```python
from build123d import *

# Parameters (mm, degrees)
BOSS_EXTRUDE1_DEPTH = 100
FILLET1_R           = 10
SKETCH4_W           = 60
SKETCH4_H           = 8
CUT_EXTRUDE1_DEPTH  = 10
FILLET2_R           = 10
SKETCH5_W           = 12
SKETCH5_H           = 14
CUT_EXTRUDE2_DEPTH  = 10
CUT_EXTRUDE3_DEPTH  = 10


with BuildPart() as part:
    # Sketch1 → Boss-Extrude1 (new body)
    with BuildSketch(Plane(origin=(0, 0, 0), x_dir=(0, 0, -1), z_dir=(1, 0, 0))):
        Polygon((0, 0), (0, 35), (11, 35), (11, 70), (19, 70), (19, 35), (40, 35), (40, 27), (8, 27), (8, 0), align=None)
    extrude(amount=-BOSS_EXTRUDE1_DEPTH)

    # Fillet1
    fillet1_edges = [part.edges().sort_by_distance(p)[0] for p in [
        (-50, 35, -11),
        (-50, 35, -19),
    ]]
    fillet(fillet1_edges, radius=FILLET1_R)

    # Sketch4 → Cut-Extrude1 (cut)
    with BuildSketch(Plane(origin=(0, 0, -40), x_dir=(-1, 0, 0), z_dir=(0, 0, -1))):
        with Locations((50, 31)):
            Rectangle(SKETCH4_W, SKETCH4_H)
    extrude(amount=-CUT_EXTRUDE1_DEPTH, mode=Mode.SUBTRACT)

    # Fillet2
    fillet2_edges = [part.edges().sort_by_distance(p)[0] for p in [
        (-20, 31, -30),
        (-80, 31, -30),
    ]]
    fillet(fillet2_edges, radius=FILLET2_R - 0.0001)  # a hair under: the kernel refuses the full size

    # Sketch5 → Cut-Extrude2 (cut)
    with BuildSketch(Plane(origin=(0, 0, -19), x_dir=(-1, 0, 0), z_dir=(0, 0, -1))):
        with Locations((20, 63)):
            Rectangle(SKETCH5_W, SKETCH5_H)
        with Locations((38, 63)):
            Rectangle(SKETCH5_W, SKETCH5_H)
        with Locations((74, 63)):
            Rectangle(SKETCH5_W, SKETCH5_H)
        with Locations((56, 63)):
            Rectangle(SKETCH5_W, SKETCH5_H)
    extrude(amount=-CUT_EXTRUDE2_DEPTH, mode=Mode.SUBTRACT)

    # Sketch6 → Cut-Extrude3 (cut)
    with BuildSketch(Plane(origin=(0, 0, -19), x_dir=(-1, 0, 0), z_dir=(0, 0, -1))):
        with BuildLine():
            Line((14, 58.578725951), (14, 56))
            ThreePointArc((14, 56), (20, 50), (26, 56))
            Line((26, 56), (26, 58.578725951))
            Line((26, 58.578725951), (14, 58.578725951))
        make_face()
        with BuildLine():
            Line((32, 56), (32, 58.578725951))
            Line((32, 58.578725951), (44, 58.578725951))
            Line((44, 58.578725951), (44, 56))
            ThreePointArc((44, 56), (38, 50), (32, 56))
        make_face()
        with BuildLine():
            Line((50, 56), (50, 58.578725951))
            Line((50, 58.578725951), (62, 58.578725951))
            Line((62, 58.578725951), (62, 56))
            ThreePointArc((62, 56), (56, 50), (50, 56))
        make_face()
        with BuildLine():
            Line((68, 56), (68, 58.578725951))
            Line((68, 58.578725951), (80, 58.578725951))
            Line((80, 58.578725951), (80, 56))
            ThreePointArc((80, 56), (74, 50), (68, 56))
        make_face()
    extrude(amount=-CUT_EXTRUDE3_DEPTH, mode=Mode.SUBTRACT)


solid = part.part
```
Source: CAD feature listing. Evaluate the final solid. Frame: model axes, mm. A direction names the side the tool comes from. Coordinates: 2 decimals unless noted, no trailing zeros. Write each loop counter-clockwise with the first axis right and the second up, starting at its lowest first coordinate (ties: lowest second). Pieces come first, ordered by that corner, then holes. Notation, with made-up numbers: (-24.5, 78.5) - (5.5, 78.5) arc R18 ccw to (5.5, 111.5) - close; hole circle Ø11 at (78, 32.5). An arc over 180 degrees is marked (long way). Answer as a JSON object with one key per item and string values.
Q1. Section query C-C, the plane z = -16.5. Output: boundary loops of the cut face in (x, y).
Ans:
{"outline": "(-100, 27) - (0, 27) - (0, 70) - (-14, 70) - (-14, 56) arc R6 cw to (-26, 56) - (-26, 70) - (-32, 70) - (-32, 56) arc R6 cw to (-44, 56) - (-44, 70) - (-50, 70) - (-50, 56) arc R6 cw to (-62, 56) - (-62, 70) - (-68, 70) - (-68, 56) arc R6 cw to (-80, 56) - (-80, 70) - (-100, 70) - close"}
Q2. Set-up query: faces 1 (the flat face through (-49, 14, -8)), 2 (the flat face through (-49, 55, -11)), 3 (the cylindrical face through (-77.15, 31.06, -33.01)), 4 (the flat face through (-50, 63, -15)). Return all of +Z, -Z, +X, -X, +Y, -Y with unobstructed straight access to the full face (end or side cutting, diameter ignored); none if empty.
Ans:
{"face 1": "-Z, +X, -X, -Y", "face 2": "+Z, +X, -X, +Y", "face 3": "-Z, +Y, -Y", "face 4": "+Z, -Z, +Y"}
Q3. Draft query along X for faces 5 (the flat face through (-90, 70, -15)), 6 (the flat face through (-80, 63, -15)), 7 (the flat face through (-44, 63, -15)). Return one class per face: released by +X, released by -X, zero draft, split by the parting line, or undercut.
Ans:
{"face 5": "zero draft", "face 6": "undercut", "face 7": "undercut"}
Q4. Section query D-D, the plane x = -38. Output: boundary loops of the cut face in (y, z).
Ans:
{"outline": "(0, -8) - (27, -8) - (27, -30) - (35, -30) - (35, -29) arc R10 cw to (45, -19) - (50, -19) - (50, -11) - (45, -11) arc R10 cw to (35, -1) - (35, 0) - (0, 0) - close"}
Q5. Section query A-A, the plane y = 65. Output: boundary loops of the cut face in (x, z).
Ans:
{"outline": "(-100, -19) - (-80, -19) - (-80, -11) - (-100, -11) - close; (-68, -19) - (-62, -19) - (-62, -11) - (-68, -11) - close; (-50, -19) - (-44, -19) - (-44, -11) - (-50, -11) - close; (-32, -19) - (-26, -19) - (-26, -11) - (-32, -11) - close; (-14, -19) - (0, -19) - (0, -11) - (-14, -11) - close"}
Q6. Section query B-B, the plane z = -34.5. Output: boundary loops of the cut face in (x, y).
Ans:
{"outline": "(-100, 27) - (-78.35, 27) - (-78.35, 35) - (-100, 35) - close; (-21.65, 27) - (0, 27) - (0, 35) - (-21.65, 35) - close"}
Q7. Material intervals for line 1 (X direction, y = 61.5, z = -18); line 2 (Z direction, x = -4, y = 24.5); line 3 (Z direction, x = -93.5, y = 62), sorted ascending. Write a range as [from, to].
Ans:
{"line 1": "x = [-100, -80], [-68, -62], [-50, -44], [-32, -26], [-14, 0]", "line 2": "z = [-8, 0]", "line 3": "z = [-19, -11]"}
Q8. First-contact query: pin 1 Ø4 at (x, z) = (-76, -28) entering from -Y; pin 2 Ø8 at (x, y) = (-49.5, 16.5) entering from -Z; pin 3 Ø5 at (x, y) = (-67, 59.5) entering from -Z. Flat tips, straight axial feed; report the tip coordinate or a pass-through.
Ans:
{"pin 1": "stops at y = 27", "pin 2": "stops at z = -8", "pin 3": "stops at z = -19"}
